from build123d import *

# Parameters (mm, degrees)
F0_W      = 177.8
F0_H      = 38.1
F1_DEPTH  = 76.2
F2_W      = 76.2
F2_H      = 66.864574
F3_DEPTH  = 38.1
F5_DEPTH  = 101.6
F6_R      = 8.255
F6_W      = 34.409892
F6_H      = 11.749721
F7_DEPTH  = 2.54
F8_W      = 69.088
F8_H      = 70.676456
F9_DEPTH  = 12.7
F10_R     = 9.097669
F11_DEPTH = 50.8
F12_R     = 7.663918
F13_DEPTH = 50.8
F14_W     = 76.2
F14_H     = 22.849783
F14_H_2   = 19.950157
F15_DEPTH = 25.4
F16_R     = 6.477
F17_DEPTH = 25.4
F18_R     = 6.477
F19_DEPTH = 25.4


with BuildPart() as f1:
    # F0 (on Right) → F1 (new body)
    with BuildSketch(Plane.YZ):
        with Locations((50.520241, -2.619057)):
            Rectangle(F0_W, F0_H)
    extrude(amount=F1_DEPTH)

    # F2 (on face) → F3 (join)
    with BuildSketch(Plane.XY.offset(16.430943)):
        with Locations((38.1, 27.691498)):
            Rectangle(F2_W, F2_H)
    extrude(amount=F3_DEPTH)

    # F4 (on face) → F5 (cut)
    with BuildSketch(Plane.YZ.offset(76.2)):
        Polygon((-5.740789, 54.530943), (-5.740789, 16.430943), (5.230976, 54.530943), align=None)
    extrude(amount=-F5_DEPTH, mode=Mode.SUBTRACT)

    # F6 (on face) → F7 (join)
    with BuildSketch(Plane.XZ.offset(38.379759)):
        with Locations((12.890441, 4.621061)):
            Circle(F6_R)
        with Locations((64.323008, 5.436914)):
            Circle(F6_R)
        with Locations((39.508564, -11.050332)):
            Rectangle(F6_W, F6_H)
    extrude(amount=F7_DEPTH)

    # F8 (on face) → F9 (cut)
    with BuildSketch(Plane.XY.offset(16.430943)):
        with Locations((38.1, 100.272013)):
            Rectangle(F8_W, F8_H)
    extrude(amount=-F9_DEPTH, mode=Mode.SUBTRACT)

    # F10 (on face) → F11 (join)
    with BuildSketch(Plane.XY.offset(3.730943)):
        with Locations((13.950241, 76.503314)):
            Circle(F10_R)
    extrude(amount=F11_DEPTH)

    # F12 (on face) → F13 (cut)
    with BuildSketch(Plane.XY.offset(54.530943)):
        with Locations((13.950241, 76.503314)):
            Circle(F12_R)
    extrude(amount=-F13_DEPTH, mode=Mode.SUBTRACT)

    # F14 (on face) → F15 (join)
    with BuildSketch(Plane(origin=(0, 0, -21.669057), x_dir=(1, 0, 0), z_dir=(0, 0, -1))):
        with Locations((38.1, -113.258853)):
            Rectangle(F14_W, F14_H)
        with Locations((38.1, 13.76035)):
            Rectangle(F14_W, F14_H_2)
    extrude(amount=F15_DEPTH)

    # F16 (on face) → F17 (join)
    with BuildSketch(Plane.YZ.offset(76.2)):
        with Locations((-13.76035, -38.966457)):
            Circle(F16_R)
        with Locations((113.258854, -38.966457)):
            Circle(F16_R)
    extrude(amount=F17_DEPTH)

    # F18 (on face) → F19 (join)
    with BuildSketch(Plane(origin=(0, 0, 0), x_dir=(0, -1, 0), z_dir=(-1, 0, 0))):
        with Locations((-113.258854, -38.966457)):
            Circle(F18_R)
        with Locations((13.76035, -38.966457)):
            Circle(F18_R)
    extrude(amount=F19_DEPTH)


solid = f1.part
The listing builds one solid part. Answer for the finished solid, in the listing's coordinates (mm). A direction names the side the tool comes from. Coordinates: 2 decimals unless noted, no trailing zeros. Write each loop counter-clockwise with the first axis right and the second up, starting at its lowest first coordinate (ties: lowest second). Pieces come first, ordered by that corner, then holes. Notation, with made-up numbers: M -25.5,-22.5 L 31.5,-22.5 A22 ccw 31.5,4.5 Z; hole C -28.75,5.25 d1. An arc over 180 degrees is marked long. Put each result on its own line as item: value. Start each with the question number.
1. A cutting plane is placed at B-B on x = 51.5. Write down the section's boundary in (y, z), then the cut area to 3 significant figures.
2. Consider line 1 (X direction, y = 128, z = 11); line 2 (X direction, y = 37, z = -15.5); line 3 (Z direction, x = 57.5, y = -18). Determine where each line is inside the solid, lowest interval first. Write a range as from..to.
3. Flat-ended cylindrical pins translate along their axes: P1, Ø14, axis at y = 83, z = 7.5, coming from the -X side; P2, Ø7.5, axis at x = 52.5, z = -37, coming from the +Y side; P3, Ø14, axis at y = 108, z = 10, coming from the +X side. Find the tip coordinate at first contact, or state that the pin passes through.
4. A cutting plane is placed at D-D on y = 9. Write down the section's boundary in (x, z), then the cut area to 3 significant figures.
5. A cutting plane is placed at A-A on z = -24. Write down the section's boundary in (x, y), then the cut area to 3 significant figures.
6. For a pull along X with two mould halves and no side action, classify faces 1 (the flat face through (-25.4, -14, -39)), 2 (the cylindrical face through (20.516, -39.632, 1.459)), 3 (the flat face through (39, -40.92, -11)) as pulls with the +X half, pulls with the -X half, needs draft (parallel to the pull), parting line crosses it, or undercut.
7. A cutting plane is placed at C-C on z = 32.5. Write down the section's boundary in (x, y).
8. Which of the six approach directions +Z, -Z, +X, -X, +Y, -Y give full straight-line access (tool end or side, diameter ignored) to faces 4 (the cylindrical face through (71.95, -39.63, 2.28)), 5 (the flat face through (38, -22, 16.431)), 6 (the cylindrical face through (88.7, 111.9, -45.3)), 7 (the flat face through (38, 64.934, 10)), 8 (the cylindrical face through (-12.522, 107.276, -41.447))?
Resolved:
1. outline: M -40.92,-16.93 L -38.38,-16.93 L -38.38,-21.67 L -23.74,-21.67 L -23.74,-47.07 L -3.79,-47.07 L -3.79,-21.67 L 101.83,-21.67 L 101.83,-47.07 L 124.68,-47.07 L 124.68,-21.67 L 139.42,-21.67 L 139.42,16.43 L 135.61,16.43 L 135.61,3.73 L 64.93,3.73 L 64.93,16.43 L 61.12,16.43 L 61.12,54.53 L 5.23,54.53 L -5.74,16.43 L -38.38,16.43 L -38.38,-5.18 L -40.92,-5.18 Z
1. area: 9,330 mm2
2. line 1: x = 0..3.56, 72.64..76.2
2. line 2: x = 0..76.2
2. line 3: z = -47.07..16.43
3. P1: stops at x = 0
3. P2: stops at y = 124.68
3. P3: stops at x = 76.2
4. outline: M 0,-21.67 L 76.2,-21.67 L 76.2,54.53 L 0,54.53 Z
4. area: 5,810 mm2
5. outline: M 0,-23.74 L 76.2,-23.74 L 76.2,-3.79 L 0,-3.79 Z; M 0,101.83 L 76.2,101.83 L 76.2,124.68 L 0,124.68 Z
5. area: 3,260 mm2
6. face 1: pulls with the -X half
6. face 2: undercut
6. face 3: needs draft
7. outline: M 0,-1.11 L 76.2,-1.11 L 76.2,61.12 L 0,61.12 Z; C 13.95,76.5 d18.2; hole C 13.95,76.5 d15.33
8. face 4: -Y
8. face 5: +Z, +X, -X, -Y
8. face 6: +X
8. face 7: +Z
8. face 8: -X
